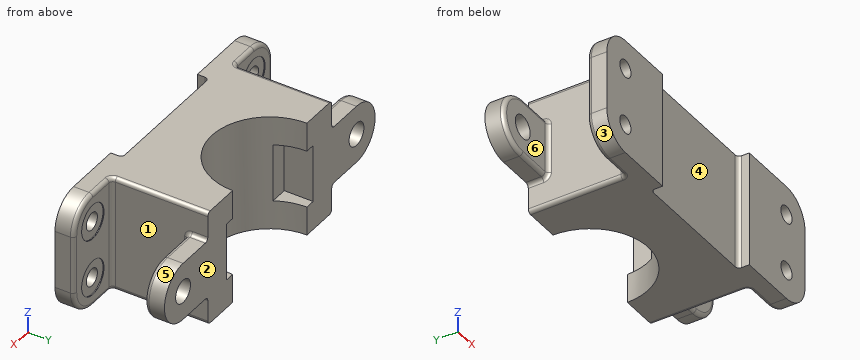
```python
from build123d import *

# Parameters (mm, degrees)
EXTRUDE_1_DEPTH             = 60
SKETCH_2_R                  = 6
EXTRUDE_2_DEPTH             = 10
FILLET_1_R                  = 15
HOLE_WIZARD_M8_1_AT_2_COUNT = 2
HOLE_WIZARD_M8_1_AT_2_PITCH = 30
HOLE_WIZARD_M8_1_AT_3_COUNT = 2
HOLE_WIZARD_M8_1_AT_3_PITCH = 130
HOLE_WIZARD_M8_1_AT_4_COUNT = 2
HOLE_WIZARD_M8_1_AT_4_PITCH = 133.416640641
FILLET_2_R                  = 2
SKETCH_5_W                  = 70
SKETCH_5_H                  = 30
CUT_EXTRUDE_1_DEPTH         = 15


with BuildPart() as part:
    # 草图1 → 凸台-拉伸1 (new body)
    with BuildSketch(Plane.XY):
        with BuildLine():
            Line((35, 0), (-35, 0))
            Line((-35, 0), (-35, -6))
            Line((-35, -6), (-80, -6))
            Line((-80, -6), (-80, 4))
            Line((-80, 4), (-50, 4))
            Line((-50, 4), (-50, 54))
            Line((-50, 54), (-30, 54))
            ThreePointArc((-30, 54), (0, 24), (30, 54))
            Line((30, 54), (50, 54))
            Line((50, 54), (50, 4))
            Line((50, 4), (80, 4))
            Line((80, 4), (80, -6))
            Line((80, -6), (35, -6))
            Line((35, -6), (35, 0))
        make_face()
    extrude(amount=-EXTRUDE_1_DEPTH)

    # 草图2 → 凸台-拉伸2 (add)
    # profile 1 of 2: a face of its own
    with BuildSketch(Plane(origin=(0, 54, 0), x_dir=(1, 0, 0), z_dir=(0, 1, 0))):
        with BuildLine():
            Line((-50, 15), (-50, 45))
            Line((-50, 45), (-70, 45))
            ThreePointArc((-70, 45), (-85, 30), (-70, 15))
            Line((-70, 15), (-50, 15))
        make_face()
        with Locations(Location((-70, 30, 0), (0, 0, 270))):
            Circle(SKETCH_2_R, mode=Mode.SUBTRACT)
    # profile 2 of 2: a face of its own
    with BuildSketch(Plane(origin=(0, 54, 0), x_dir=(1, 0, 0), z_dir=(0, 1, 0))):
        with BuildLine():
            Line((50, 45), (70, 45))
            ThreePointArc((70, 45), (85, 30), (70, 15))
            Line((70, 15), (50, 15))
            Line((50, 15), (50, 45))
        make_face()
        with Locations(Location((70, 30, 0), (0, 0, 90))):
            Circle(SKETCH_2_R, mode=Mode.SUBTRACT)
    extrude(amount=-EXTRUDE_2_DEPTH)

    # 圆角1
    fillet_1_edges = [part.edges().sort_by_distance(p)[0] for p in [
        (-80, -1, 0),
        (80, -1, 0),
        (80, -1, -60),
        (-80, -1, -60),
    ]]
    fillet(fillet_1_edges, radius=FILLET_1_R)

    # 草图4 → M8 六角头螺栓的柱形沉头孔1 (revolve, cut)
    with BuildSketch(Plane(origin=(-65, 4, -15), x_dir=(0, 0, 1), z_dir=(1, 0, 0))):
        Polygon((0, 0), (0, 10), (4.5, 10), (4.5, 0.5), (9, 0.5), (9, 0.020977491), (9.025, 0), align=None)
    hole_wizard_m8_1 = revolve(axis=Axis((-65, 10.35, -15), (0, -1, 0)), mode=Mode.SUBTRACT)

    # M8 六角头螺栓的柱形沉头孔1 at 2: M8 六角头螺栓的柱形沉头孔1 ×2
    with Locations(*[(0, 0, -i * HOLE_WIZARD_M8_1_AT_2_PITCH) for i in range(1, HOLE_WIZARD_M8_1_AT_2_COUNT)]):
        add(hole_wizard_m8_1, mode=Mode.SUBTRACT)

    # M8 六角头螺栓的柱形沉头孔1 at 3: M8 六角头螺栓的柱形沉头孔1 ×2
    with Locations(*[(i * HOLE_WIZARD_M8_1_AT_3_PITCH, 0, 0) for i in range(1, HOLE_WIZARD_M8_1_AT_3_COUNT)]):
        add(hole_wizard_m8_1, mode=Mode.SUBTRACT)

    # M8 六角头螺栓的柱形沉头孔1 at 4: M8 六角头螺栓的柱形沉头孔1 ×2
    with Locations(*[Vector(0.9743911956946198, 0, -0.22485950669875843) * (i * HOLE_WIZARD_M8_1_AT_4_PITCH) for i in range(1, HOLE_WIZARD_M8_1_AT_4_COUNT)]):
        add(hole_wizard_m8_1, mode=Mode.SUBTRACT)

    # 圆角2
    fillet_2_edges = [part.edges().sort_by_distance(p)[0] for p in [
        (-57.5, 4, 0),
        (-50, 29, 0),
        (50, 29, 0),
        (-50, 4, -30),
        (50, 4, -30),
        (35, 0, -30),
        (-35, 0, -30),
        (50, 29, -60),
        (-60, 44, -15),
        (-50, 49, -15),
        (-85, 44, -30),
        (-60, 44, -45),
        (-50, 44, -30),
        (-50, 49, -45),
        (-50, 29, -60),
        (-57.5, 4, -60),
        (85, 44, -30),
        (60, 44, -15),
        (50, 44, -30),
        (50, 49, -15),
        (60, 44, -45),
        (50, 49, -45),
        (80, 4, -30),
        (57.5, 4, 0),
        (57.5, 4, -60),
        (75.606601718, 4, -4.393398282),
        (75.606601718, 4, -55.606601718),
        (-80, 4, -30),
        (-75.606601718, 4, -4.393398282),
        (-75.606601718, 4, -55.606601718),
    ]]
    fillet(fillet_2_edges, radius=FILLET_2_R)

    # 草图5 → 切除-拉伸1 (cut)
    with BuildSketch(Plane(origin=(0, 54, 0), x_dir=(1, 0, 0), z_dir=(0, 1, 0))):
        with Locations((0, 30)):
            Rectangle(SKETCH_5_W, SKETCH_5_H)
    extrude(amount=-CUT_EXTRUDE_1_DEPTH, mode=Mode.SUBTRACT)


solid = part.part
```
Part model, mm, in its own coordinate system. Face numbers are marked on the shaded views. A direction names the side the tool comes from. Round coordinates to 2 decimals unless told otherwise and drop trailing zeros. Write each loop counter-clockwise with the first axis right and the second up, starting at its lowest first coordinate (ties: lowest second). Pieces come first, ordered by that corner, then holes. Notation, with made-up numbers: M 38,44 L 90,44 A13 cw 90,64 Z; hole C 24.5,-9.75 d9. An arc over 180 degrees is marked long. Answer as CSV lines item,"result". Start each with the question number.
1) Drill centre lines: L1, parallel to Z at x = -65, y = -1; L2, parallel to Y at x = -77, z = -26; L3, parallel to X at y = 40, z = -22. Where is each one in solid material? Low to high.
2) Which spindle directions (+Z, -Z, +X, -X, +Y, -Y) get a long thin tool onto all of the face, cutting with end or side? Do the marked faces 4, 5 and 6. Say none if no direction does.
3) Band-saw the part on C-C (y = 34). List the corners of the cut face in (x, z).
4) Band-saw the part on A-A (y = 22). List the corners of the cut face in (x, z).
5) Band-saw the part on B-B (z = -30). Count the separate pieces of the cut face and the enclosed holes in it, then the cut area to 3 significant figures.
6) Band-saw the part on D-D (x = 0). List the corners of the cut face in (y, z), then the cut area to 3 significant figures.
7) Drop flat-ended pins along their axis: pin 1 (2 mm diameter, centred on y = -3.5, z = -25, fed in from +X); pin 2 (9 mm diameter, centred on x = 60.5, y = 50, fed in from -Z); pin 3 (7.5 mm diameter, centred on y = 44.5, z = -23, fed in from -X). Give the stop position or say it passes through.
8) Mould opens along Y. For the marked faces 1, 2 and 3 say: +Y half, -Y half, draft (parallel to the pull), parting line (faces both ways), or undercut.
Worked out:
1,L1,"-60 to -49.5, -40.5 to -19.5, -10.5 to 0"
1,L2,"-6 to 4, 44 to 54"
1,L3,"-50 to -35, 35 to 50"
2,face 4,"+Z, -Z, -Y"
2,face 5,"+X, +Y"
2,face 6,"+Z, -Z, -X"
3,outline,"M -50,-58 A2 ccw -48,-60 L -22.36,-60 L -22.36,0 L -48,0 A2 ccw -50,-2 Z; M 22.36,-60 L 48,-60 A2 ccw 50,-58 L 50,-2 A2 ccw 48,0 L 22.36,0 Z"
4,outline,"M -50,-58 A2 ccw -48,-60 L 48,-60 A2 ccw 50,-58 L 50,-2 A2 ccw 48,0 L -48,0 A2 ccw -50,-2 Z"
5,separate pieces,"3"
5,enclosed holes,"0"
5,area,"5,040 mm²"
6,outline,"M 0,-60 L 24,-60 L 24,0 L 0,0 Z"
6,area,"1,440 mm²"
7,pin 1,"x = 80"
7,pin 2,"z = -45"
7,pin 3,"x = -84.58"
8,face 1,"undercut"
8,face 2,"+Y half"
8,face 3,"draft"
